```python
from build123d import *

# Parameters (mm, degrees)
PAD_DEPTH   = 8.5
FILLET_R    = 1.2
FILLET001_R = 1


with BuildPart() as part:
    # Sketch → Pad (new body)
    with BuildSketch(Plane.XY):
        Polygon((0, 0), (0, 12), (42, 12), (42, 9), (42, 9), (42, 3), (48, 3), (48, 0), align=None)
    extrude(amount=PAD_DEPTH)

    # Fillet
    fillet_edges = [part.edges().sort_by_distance(p)[0] for p in [
        (48, 0, 4.25),
        (48, 3, 4.25),
        (42, 3, 4.25),
        (42, 12, 4.25),
        (0, 12, 4.25),
        (0, 0, 4.25),
    ]]
    fillet(fillet_edges, radius=FILLET_R)

    # Fillet001
    fillet001_edges = [part.edges().sort_by_distance(p)[0] for p in [
        (21, 12, 8.5),
        (21, 12, 0),
    ]]
    fillet(fillet001_edges, radius=FILLET001_R)


solid = part.part
```
Here's how the part is built. I have some questions about the finished solid (model axes, mm). A direction names the side the tool comes from. Give positions to 0.01 mm unless a question says otherwise; leave off trailing zeros. Order: outer loops, then holes, each group sorted by start corner. A loop starts at its lowest first (then second) coordinate and runs counter-clockwise, first axis right, second up. Notation, with made-up numbers: M 19,-10.5 L 29,-10.5 A18 cw 29,23.5 Z; hole C 81,85 d2. An arc over 180 degrees is marked long. Use a Markdown table: item, result. Add a question column.
1. Suppose I cut it at A-A (y = 9.25). List the corners of the cut face in (x, z) for me.
2. On a 3-axis mill with a long thin cutter (end or side, diameter ignored), from which of +Z, -Z, +X, -X, +Y, -Y can I reach the whole of each face in a straight line? I mean faces 1 (the cylindrical face through (45.025, 2.699, 0.285)), 2 (the cylindrical face through (41.699, 7.454, 8.215)), 3 (the flat face through (0, 6, 4)). Say none if no direction works.
3. For pin 1 Ø1.8 at (x, z) = (45.5, 6) entering from +Y; pin 2 Ø2 at (y, z) = (8.5, 3) entering from +X, each with a flat end and sliding along its axis, tell me the tip position at first contact or that it passes through.
4. Suppose I cut it at B-B (z = 6). List the corners of the cut face in (x, y) for me, and give its area (3 significant figures).
5. I need wall thicknesses on probe 1 along X at (y, z) = (6.75, 1.25); probe 2 along Z at (x, y) = (41.5, 6.75); probe 3 along X at (y, z) = (0.75, 1.25). Which ranges of each line are inside material? Lowest first, please. Write a range as from..to.
Results list:
| question | item | result |
|---|---|---|
| 1 | outline | M 0,1 A1 ccw 1,0 L 41,0 A1 ccw 42,1 L 42,7.5 A1 ccw 41,8.5 L 1,8.5 A1 ccw 0,7.5 Z |
| 2 | face 1 | -Z, +X, +Y |
| 2 | face 2 | +Z, +X, +Y |
| 2 | face 3 | +Z, -Z, -X, +Y, -Y |
| 3 | pin 1 | stops at y = 3 |
| 3 | pin 2 | stops at x = 42 |
| 4 | outline | M 0,1.2 A1.2 ccw 1.2,0 L 46.8,0 A1.2 ccw 48,1.2 L 48,1.8 A1.2 ccw 46.8,3 L 43.2,3 A1.2 cw 42,4.2 L 42,10.8 A1.2 ccw 40.8,12 L 1.2,12 A1.2 ccw 0,10.8 Z |
| 4 | area | 521 mm² |
| 5 | probe 1 | x = 0..42 |
| 5 | probe 2 | z = 0.13..8.37 |
| 5 | probe 3 | x = 0.09..47.91 |
